from build123d import *

# Parameters (mm, degrees)
F1_DEPTH = 340
F2_R     = 250
F4_DEPTH = 277.5


with BuildPart() as f1:
    # F0 (on Front) → F1 (new body)
    with BuildSketch(Plane.XZ):
        with BuildLine():
            Line((0, 450), (0, 0))
            Line((0, 0), (500, 0))
            Line((500, 0), (500, 100))
            Line((500, 100), (250, 100))
            ThreePointArc((250, 100), (143.933983, 143.933983), (100, 250))
            Line((100, 250), (100, 450))
            Line((100, 450), (0, 450))
        make_face()
    extrude(amount=-F1_DEPTH)

    # F2
    f2_edges = [f1.edges().sort_by_distance(p)[0] for p in [
        (500, 0, 50),
    ]]
    fillet(f2_edges, radius=F2_R)

    # F3 (on face) → F4 (cut)
    with BuildSketch(Plane.YZ.offset(100)):
        with BuildLine():
            Line((50, 450), (50, 300))
            ThreePointArc((50, 300), (57.132359, 271.627257), (76.833752, 250))
            Line((76.833752, 250), (143.166248, 250))
            ThreePointArc((143.166248, 250), (162.867641, 271.627257), (170, 300))
            Line((170, 300), (170, 450))
            Line((170, 450), (50, 450))
        make_face()
    extrude(amount=-F4_DEPTH, mode=Mode.SUBTRACT)


solid = f1.part
Input: part model. Units: mm. Frame: model coordinates. A direction names the side the tool comes from. Coordinates: 2 decimals unless noted, no trailing zeros. Loops run counter-clockwise (first coordinate to the right, second up) from the corner with the lowest first, then second, coordinate; pieces in that order, holes last. Notation, with made-up numbers: (74, 22) -> (117, 22) arc R16 cw to (117, 34) -> close; hole circle Ø3 at (53.5, -35). An arc over 180 degrees is marked (long way). Write item = value, one per line. Start each with the question number.
Item 1: Cut plane D-D, the plane y = 24.5. Return loops of the section in (x, z).
Item 2: Reachability of faces 1 (the face through (50.7, 162.67, 271.26)), 2 (the face through (95, 0, 178)), 3 (the face through (100, 262, 349)) from +Z, -Z, +X, -X, +Y, -Y: full face, straight path, thin tool, end or side. Return the list, or none.
Item 3: Cut plane B-B, the plane x = 72.5. Return loops of the section in (y, z), plus the area to 3 significant figures.
Item 4: First-contact query: P1, Ø6, axis at y = 305, z = 403, coming from the +X side. Flat tip, straight axial feed; report the tip coordinate or a pass-through.
Item 5: Cut plane A-A, the plane z = 405. Return loops of the section in (x, y).
Item 6: Cut plane C-C, the plane y = 257. Return loops of the section in (x, z), plus the area to 3 significant figures.
Item 7: Material intervals for line 1 (Y direction, x = 43.5, z = 426); line 2 (X direction, y = 20, z = 372), sorted ascending.
Item 8: Mould query, pull axis Y, two halves, no side actions, for faces 4 (the face through (377, 205, 100)), 5 (the face through (50.7, 56.94, 271.99)), 6 (the face through (135, 340, 128)). Classes: pulls with the +Y half, pulls with the -Y half, needs draft (parallel to the pull), parting line crosses it, or undercut.
Ans:
q1.outline = (0, 0) -> (357.93, 0) -> (357.93, 100) -> (250, 100) arc R150 cw to (100, 250) -> (100, 450) -> (0, 450) -> close
q2.face_1 = +Z, +X, -X
q2.face_2 = +Z, -Z, +X, -X, -Y
q2.face_3 = +Z, +X, +Y, -Y
q3.outline = (0, 0) -> (340, 0) -> (340, 450) -> (170, 450) -> (170, 300) arc R60 cw to (143.17, 250) -> (76.83, 250) arc R60 cw to (50, 300) -> (50, 450) -> (0, 450) -> close
q3.area = 130,000 mm²
q4.P1 = 100
q5.outline = (0, 0) -> (100, 0) -> (100, 50) -> (0, 50) -> close; (0, 170) -> (100, 170) -> (100, 340) -> (0, 340) -> close
q6.outline = (0, 0) -> (500, 0) -> (500, 100) -> (250, 100) arc R150 cw to (100, 250) -> (100, 450) -> (0, 450) -> close
q6.area = 89,800 mm²
q7.line_1 = 0 to 50, 170 to 340
q7.line_2 = 0 to 100
q8.face_4 = needs draft
q8.face_5 = undercut
q8.face_6 = pulls with the +Y half
